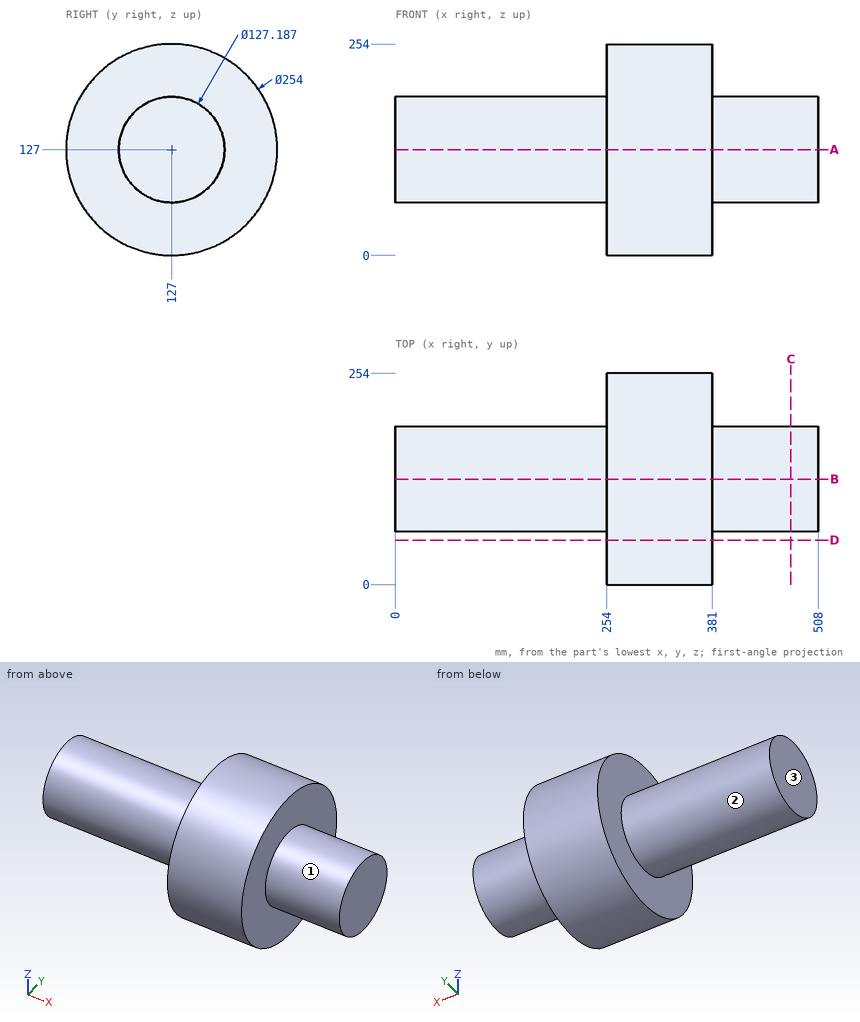
Job drawing, mm, ordinate dimensions from the low corner. One solid piece. A direction names the side the tool comes from. Coordinates: 2 decimals unless noted, no trailing zeros. Write each loop counter-clockwise with the first axis right and the second up, starting at its lowest first coordinate (ties: lowest second). Pieces come first, ordered by that corner, then holes.
Item 1: Slice it at D-D (y = 53.5). Write the cut outline in (x, z), and give its area (3 significant figures).
Item 2: Pin check, flat tips, straight feed: pin 1 (12 mm diameter, centred on y = 57.5, z = 224.5, fed in from +X); pin 2 (5 mm diameter, centred on x = 225, y = 185, fed in from +Z); pin 3 (6 mm diameter, centred on x = 102.5, y = 137, fed in from +Z); pin 4 (8 mm diameter, centred on x = 222.5, z = 55.5, fed in from -Y). Stop position of each tip, or through.
Item 3: Slice it at C-C (x = 475.5). Write the cut outline in (y, z), and give its area (3 significant figures).
Item 4: Which spindle directions (+Z, -Z, +X, -X, +Y, -Y) get a long thin tool onto all of the face, cutting with end or side? Do the marked faces 1, 2 and 3. Say none if no direction does.
Item 5: Slice it at A-A (z = 127). Write the cut outline in (x, y), and give its area (3 significant figures).
Item 6: Probe line 1 (X direction, y = 185, z = 100.5); line 2 (Z direction, x = 368.5, y = 122); line 3 (Z direction, x = 293.5, y = 56.5) (1 decimal). List the from-to ranges inside material, lowest first.
Results found:
1. outline: (254, 23.43) - (381, 23.43) - (381, 230.57) - (254, 230.57) - close
1. area: 26,300 mm2
2. pin 1: stops at x = 381
2. pin 2: stops at z = 158.05
2. pin 3: stops at z = 190.21
2. pin 4: passes through
3. outline: circle Ø127.19 at (127, 127)
3. area: 12,700 mm2
4. face 1: +X
4. face 2: -X
4. face 3: +Z, -Z, -X, +Y, -Y
5. outline: (0, 63.41) - (254, 63.41) - (254, 0) - (381, 0) - (381, 63.41) - (508, 63.41) - (508, 190.59) - (381, 190.59) - (381, 254) - (254, 254) - (254, 190.59) - (0, 190.59) - close
5. area: 80,700 mm2
6. line 1: x = 254 to 381
6. line 2: z = 0.1 to 253.9
6. line 3: z = 21.4 to 232.6
